Geometry: final body of the model. Coordinates: model frame, mm. Face numbers are marked on the shaded views. A direction names the side the tool comes from. Coordinates: 2 decimals unless noted, no trailing zeros. Loops run counter-clockwise (first coordinate to the right, second up) from the corner with the lowest first, then second, coordinate; pieces in that order, holes last. Notation, with made-up numbers: (41.5, 68) - (76.5, 68) arc R14 ccw to (76.5, 74) - close; hole circle Ø9 at (81.5, 38.5). An arc over 180 degrees is marked (long way). Return JSON: item names as keys, results as strings.
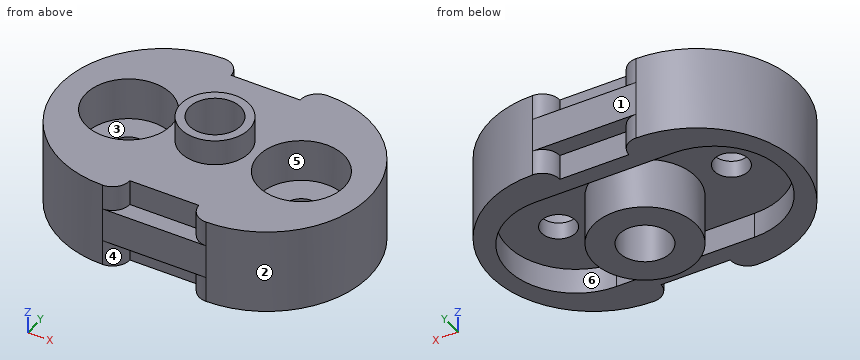
from build123d import *

# Parameters (mm, degrees)
BOSS_EXTRUDE1_DEPTH = 10
BOSS_EXTRUDE2_DEPTH = 7.5
BOSS_EXTRUDE3_DEPTH = 7.5
CUT_EXTRUDE1_DEPTH  = 7.5
SKETCH5_R           = 12.5
CUT_EXTRUDE3_DEPTH  = 12.5
SKETCH6_R           = 5
CUT_EXTRUDE4_DEPTH  = 17.5
SKETCH7_R           = 10
BOSS_EXTRUDE4_DEPTH = 7.5
SKETCH8_R           = 7.5
CUT_EXTRUDE5_DEPTH  = 25
SKETCH10_R          = 15
BOSS_EXTRUDE6_DEPTH = 15
SKETCH11_R          = 7.5
CUT_EXTRUDE6_DEPTH  = 20


with BuildPart() as part:
    # Sketch1 → Boss-Extrude1 (new body)
    with BuildSketch(Plane.XY):
        with BuildLine():
            Line((-30, 60), (0, 60))
            ThreePointArc((0, 60), (30, 30), (0, 0))
            Line((0, 0), (-30, 0))
            ThreePointArc((-30, 0), (-60, 30), (-30, 60))
        make_face()
    extrude(amount=BOSS_EXTRUDE1_DEPTH)

    # Sketch2 → Boss-Extrude2 (add)
    with BuildSketch(Plane.XY.offset(10)):
        with BuildLine():
            Line((-25, 55), (-5, 55))
            ThreePointArc((-5, 55), (-3.535533906, 58.535533906), (0, 60))
            ThreePointArc((0, 60), (30, 30), (0, 0))
            ThreePointArc((0, 0), (-3.535533906, 1.464466094), (-5, 5))
            Line((-5, 5), (-25, 5))
            ThreePointArc((-25, 5), (-26.464466094, 1.464466094), (-30, 0))
            ThreePointArc((-30, 0), (-60, 30), (-30, 60))
            ThreePointArc((-30, 60), (-26.464466094, 58.535533906), (-25, 55))
        make_face()
    extrude(amount=BOSS_EXTRUDE2_DEPTH)

    # Sketch3 → Boss-Extrude3 (add)
    with BuildSketch(Plane(origin=(0, 0, 0), x_dir=(-1, 0, 0), z_dir=(0, 0, -1))):
        with BuildLine():
            Line((5, 55), (25, 55))
            ThreePointArc((25, 55), (26.464466094, 58.535533906), (30, 60))
            ThreePointArc((30, 60), (60, 30), (30, 0))
            ThreePointArc((30, 0), (26.464466094, 1.464466094), (25, 5))
            Line((25, 5), (5, 5))
            ThreePointArc((5, 5), (3.535533906, 1.464466094), (0, 0))
            ThreePointArc((0, 0), (-30, 30), (0, 60))
            ThreePointArc((0, 60), (3.535533906, 58.535533906), (5, 55))
        make_face()
    extrude(amount=BOSS_EXTRUDE3_DEPTH)

    # Sketch4 → Cut-Extrude1 (cut)
    with BuildSketch(Plane(origin=(0, 0, -7.5), x_dir=(-1, 0, 0), z_dir=(0, 0, -1))):
        with BuildLine():
            Line((-5, 50), (35, 50))
            ThreePointArc((35, 50), (55, 30), (35, 10))
            Line((35, 10), (-5, 10))
            ThreePointArc((-5, 10), (-25, 30), (-5, 50))
        make_face()
    extrude(amount=-CUT_EXTRUDE1_DEPTH, mode=Mode.SUBTRACT)

    # Sketch5 → Cut-Extrude3 (cut)
    with BuildSketch(Plane.XY.offset(17.5)):
        with Locations((10, 30)):
            Circle(SKETCH5_R)
        with Locations((-40, 30)):
            Circle(SKETCH5_R)
    extrude(amount=-CUT_EXTRUDE3_DEPTH, mode=Mode.SUBTRACT)

    # Sketch6 → Cut-Extrude4 (cut)
    with BuildSketch(Plane.XY.offset(5)):
        with Locations((10, 30)):
            Circle(SKETCH6_R)
        with Locations((-40, 30)):
            Circle(SKETCH6_R)
    extrude(amount=-CUT_EXTRUDE4_DEPTH, mode=Mode.SUBTRACT)

    # Sketch7 → Boss-Extrude4 (add)
    with BuildSketch(Plane.XY.offset(17.5)):
        with Locations((-15, 30)):
            Circle(SKETCH7_R)
    extrude(amount=BOSS_EXTRUDE4_DEPTH)

    # Sketch8 → Cut-Extrude5 (cut)
    with BuildSketch(Plane.XY.offset(25)):
        with Locations((-15, 30)):
            Circle(SKETCH8_R)
    extrude(amount=-CUT_EXTRUDE5_DEPTH, mode=Mode.SUBTRACT)

    # Sketch10 → Boss-Extrude6 (add)
    with BuildSketch(Plane(origin=(0, 0, 0), x_dir=(-1, 0, 0), z_dir=(0, 0, -1))):
        with Locations((15, 30)):
            Circle(SKETCH10_R)
    extrude(amount=BOSS_EXTRUDE6_DEPTH)

    # Sketch11 → Cut-Extrude6 (cut)
    with BuildSketch(Plane(origin=(0, 0, -15), x_dir=(-1, 0, 0), z_dir=(0, 0, -1))):
        with Locations((15, 30)):
            Circle(SKETCH11_R)
    extrude(amount=-CUT_EXTRUDE6_DEPTH, mode=Mode.SUBTRACT)


solid = part.part
Item 1: Ray query, probe 1 along X at (y, z) = (27, 7.5); probe 2 along Z at (x, y) = (21.5, 15); probe 3 along Z at (x, y) = (-45, 33.5). Return the intervals inside material, ascending. Write a range as from..to.
Worked out:
{"probe 1": "-59.85..-52.13, -27.87..-21.87, -8.13..-2.13, 22.13..29.85", "probe 2": "-7.5..17.5", "probe 3": "0..5"}
Item 2: Section query D-D, the plane x = 2.5. Return loops of the section in (y, z), and give its area (3 significant figures).
Worked out:
{"outline": "(0.1, -7.5) - (10, -7.5) - (10, 0) - (50, 0) - (50, -7.5) - (59.9, -7.5) - (59.9, 17.5) - (40, 17.5) - (40, 5) - (20, 5) - (20, 17.5) - (0.1, 17.5) - close", "area": "945 mm^2"}
Item 3: First-contact query: pin 1 Ø4 at (x, z) = (2.5, -10) entering from -Y; pin 2 Ø12 at (y, z) = (14, 10) entering from -X; pin 3 Ø6 at (x, z) = (-14, 13.5) entering from -Y; pin 4 Ø5.5 at (x, y) = (-17.5, 58.5) entering from -Z. Flat tips, straight axial feed; report the tip coordinate or a pass-through.
Worked out:
{"pin 1": "through", "pin 2": "x = -58.28", "pin 3": "y = 5", "pin 4": "z = 0"}
Item 4: Section query A-A, the plane x = -15. Return loops of the section in (y, z).
Worked out:
{"outline": "(0, 0) - (5, 0) - (5, -7.5) - (10, -7.5) - (10, 0) - (15, 0) - (15, -15) - (22.5, -15) - (22.5, 25) - (20, 25) - (20, 17.5) - (5, 17.5) - (5, 10) - (0, 10) - close; (37.5, -15) - (45, -15) - (45, 0) - (50, 0) - (50, -7.5) - (55, -7.5) - (55, 0) - (60, 0) - (60, 10) - (55, 10) - (55, 17.5) - (40, 17.5) - (40, 25) - (37.5, 25) - close"}
Item 5: Mould query, pull axis Y, two halves, no side actions, for the marked faces 1, 2 and 3. Classes: +Y half, -Y half, draft (parallel to the pull), parting line (faces both ways), or undercut.
Worked out:
{"face 1": "+Y half", "face 2": "parting line", "face 3": "undercut"}
Item 6: Section query C-C, the plane y = 13.5. Return loops of the section in (x, z), and give its area (3 significant figures).
Worked out:
{"outline": "(-55.05, -7.5) - (-46.3, -7.5) - (-46.3, 0) - (16.3, 0) - (16.3, -7.5) - (25.05, -7.5) - (25.05, 17.5) - (-55.05, 17.5) - close", "area": "1,530 mm^2"}
Item 7: Section query B-B, the plane z = 13. Return loops of the section in (x, y).
Worked out:
{"outline": "(-30, 0) arc R5 ccw to (-25, 5) - (-5, 5) arc R5 ccw to (0, 0) arc R30 ccw to (0, 60) arc R5 ccw to (-5, 55) - (-25, 55) arc R5 ccw to (-30, 60) arc R30 ccw to start; hole circle Ø25 at (-40, 30); hole circle Ø15 at (-15, 30); hole circle Ø25 at (10, 30)"}
Item 8: Reachability of the marked faces 4, 5 and 6 from +Z, -Z, +X, -X, +Y, -Y: full face, straight path, thin tool, end or side. Return the list, or none.
Worked out:
{"face 4": "-Z, -Y", "face 5": "+Z", "face 6": "-Z"}
